Geometry check sheet. Reference: the model listing, model coordinates, mm. A direction names the side the tool comes from. Coordinates: 2 decimals unless noted, no trailing zeros. Loops run counter-clockwise (first coordinate to the right, second up) from the corner with the lowest first, then second, coordinate; pieces in that order, holes last. Notation, with made-up numbers: M 31,-33.75 L 59,-33.75 A19 ccw 59,-14.75 Z; hole C 4,42.5 d2. An arc over 180 degrees is marked long. One line per question, with ' | ' between items. Start each with the question number.
from build123d import *

# Parameters (mm, degrees)
CONG_1_R                             = 0.2
ENL_VEMENT_START                     = -0.515
ENL_VEMENT_DE_MATI_RE_LISSAGE1_DEPTH = 1.03
R_P_TITION_CIRCULAIRE1_COUNT         = 2
R_P_TITION_CIRCULAIRE1_ANGLE         = 90
CHANFREIN1_SIZE                      = 0.5


# Read off the part's stored shape, not the designer's step: Enlèvement de matière-Lissage1
with BuildPart() as part:
    # Esquisse1 → Révolution1 (revolve)
    with BuildSketch(Plane.XY, mode=Mode.PRIVATE) as r_volution1_sk:
        with BuildLine():
            Line((3.15, 2.5), (3.15, 4.05))
            Line((3.15, 4.05), (1.592505731, 4.05))
            ThreePointArc((1.592505731, 4.05), (1.431705614, 4.012092102), (1.304769911, 3.906351792))
            ThreePointArc((1.304769911, 3.906351792), (0.334815673, 2.059247972), (0, 0))
            Line((0, 0), (19.15, 0))
            Line((19.15, 0), (19.15, 2.5))
            Line((19.15, 2.5), (3.15, 2.5))
        make_face()
    revolve(r_volution1_sk.sketch.rotate(Axis((-25.4, 0, 0), (1, 0, 0)), 90), axis=Axis((-25.4, 0, 0), (1, 0, 0)))

    # Congé1
    cong_1_edges = [part.edges().sort_by_distance(p)[0] for p in [
        (3.15, 0, -2.5),
    ]]
    fillet(cong_1_edges, radius=CONG_1_R)

    # Enlèvement de matière-Lissage1 outline → Enlèvement de matière-Lissage1 (cut)
    with BuildSketch(Plane.XY.offset(ENL_VEMENT_START)):
        Polygon((2.34, -0.983319232), (2.34, 0.983319232), (0.349683815, 2.103238481), (-1, 2.862684089), (-1, -2.862684089), (0.349683815, -2.103238481), align=None)
    enl_vement_de_mati_re_lissage1 = extrude(amount=ENL_VEMENT_DE_MATI_RE_LISSAGE1_DEPTH, mode=Mode.SUBTRACT)

    # Répétition circulaire1: Enlèvement de matière-Lissage1 ×2 about axis
    r_p_tition_circulaire1_axis = Axis((0, 0, 0), (-1, 0, 0))
    for i in range(1, R_P_TITION_CIRCULAIRE1_COUNT):
        add(enl_vement_de_mati_re_lissage1.rotate(r_p_tition_circulaire1_axis, i * R_P_TITION_CIRCULAIRE1_ANGLE / (R_P_TITION_CIRCULAIRE1_COUNT - 1)), mode=Mode.SUBTRACT)

    # Esquisse4 → Enlèvement de matière-Révolution1 (revolve, cut)
    with BuildSketch(Plane.XY, mode=Mode.PRIVATE) as enl_vement_de_mati_re_r_volution1_sk:
        Polygon((0, 0), (0, 1.01462874), (2.34, 0.851), (2.616506661, 0), align=None)
    revolve(enl_vement_de_mati_re_r_volution1_sk.sketch.rotate(Axis((-3.175, 0, 0), (1, 0, 0)), 13.8231891), axis=Axis((-3.175, 0, 0), (1, 0, 0)), mode=Mode.SUBTRACT)

    # Chanfrein1
    chanfrein1_edges = [part.edges().sort_by_distance(p)[0] for p in [
        (19.15, 0, -2.5),
    ]]
    chamfer(chanfrein1_edges, length=CHANFREIN1_SIZE)


solid = part.part
1. Depth check by flat-ended pin: pin 1 Ø3 at (x, y) = (9.5, 3) entering from -Z; pin 2 Ø1.6 at (x, z) = (1, -1.5) entering from +Y; pin 3 Ø2 at (y, z) = (3, -3) entering from -X; pin 4 Ø4 at (y, z) = (2, 1.5) entering from +X. Enter the tip coordinate at first touch or a pass-through.
2. Sectioned sample at A-A (x = 8.25). Record the cut outline in (y, z).
3. Tool access check on faces 1 (the flat face through (3.15, 1, -3)), 2 (the flat face through (1, 1, 0.515)). Record the directions out of +Z, -Z, +X, -X, +Y, -Y that give a thin tool (end or side, any length) a straight path to the whole face; none if there is none.
4. Draft check along Z on faces 3 (the flat face through (19.15, 0, 0)), 4 (the flat face through (1.33, -0.01, 1.55)), 5 (the cylindrical face through (2.36, 3.954, -0.878)). Enter one of: +Z half, -Z half, draft (parallel to the pull), parting line (faces both ways), or undercut.
5. Thickness scan on line 1 (Y direction, x = 8.75, z = 1.5); line 2 (Y direction, x = 5, z = 0); line 3 (X direction, y = 1, z = -2.5). Record the ranges inside material, lowest first.
Result:
1) pin 1: stops at z = -2 | pin 2: stops at y = 3.94 | pin 3: stops at x = 0.87 | pin 4: stops at x = 19.15
2) outline: C 0,0 d5
3) face 1: +X | face 2: -X
4) face 3: draft | face 4: undercut | face 5: parting line
5) line 1: y = -2 to 2 | line 2: y = -2.5 to 2.5 | line 3: x = 0.58 to 3.15
